Study the drawing (mm; zero at the part's minimum x, y, z) and answer. Give positions to 0.01 mm unless a question says otherwise; leave off trailing zeros. Order: outer loops, then holes, each group sorted by start corner. A loop starts at its lowest first (then second) coordinate and runs counter-clockwise, first axis right, second up. Notation, with made-up numbers: (14.25, 20.5) - (41.25, 20.5) arc R8 cw to (41.25, 31.5) - close; hole circle Ø6 at (89, 33.5). An arc over 180 degrees is marked (long way). Return JSON: item names as keys, results as strings.
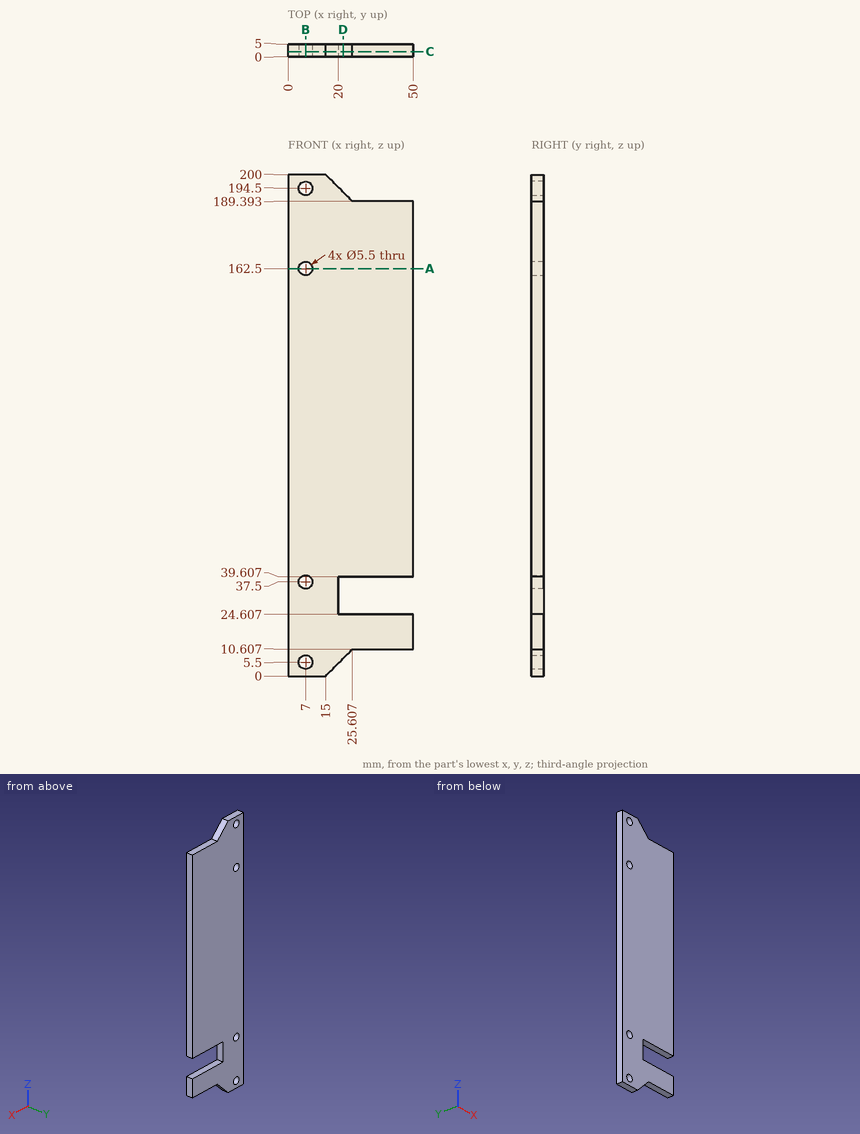
Q1. A cutting plane is placed at C-C (y = 2). Write down the section's boundary in (x, z).
Values:
{"outline": "(0, 0) - (15, 0) - (25.61, 10.61) - (50, 10.61) - (50, 24.61) - (20, 24.61) - (20, 39.61) - (50, 39.61) - (50, 189.39) - (25.61, 189.39) - (15, 200) - (0, 200) - close; hole circle Ø5.5 at (7, 5.5); hole circle Ø5.5 at (7, 37.5); hole circle Ø5.5 at (7, 162.5); hole circle Ø5.5 at (7, 194.5)"}
Q2. Given pin 1 (5 mm diameter, centred on x = 7, z = 5.5, fed in from +Y), flat-ended and moving along its own axis, determine where the tip first touches the part or whether it passes through.
Values:
{"pin 1": "passes through"}
Q3. A cutting plane is placed at A-A (z = 162.5). Write down the section's boundary in (x, y).
Values:
{"outline": "(0, 0) - (4.25, 0) - (4.25, 5) - (0, 5) - close; (9.75, 0) - (50, 0) - (50, 5) - (9.75, 5) - close"}
Q4. A cutting plane is placed at B-B (x = 7). Write down the section's boundary in (y, z).
Values:
{"outline": "(0, 0) - (5, 0) - (5, 2.75) - (0, 2.75) - close; (0, 8.25) - (5, 8.25) - (5, 34.75) - (0, 34.75) - close; (0, 40.25) - (5, 40.25) - (5, 159.75) - (0, 159.75) - close; (0, 165.25) - (5, 165.25) - (5, 191.75) - (0, 191.75) - close; (0, 197.25) - (5, 197.25) - (5, 200) - (0, 200) - close"}
Q5. Consider L1, parallel to Z at x = 37.5, y = 3.95; L2, parallel to X at y = 2.6, z = 37.5; L3, parallel to Z at x = 5, y = 3.15 (1 decimal). Determine where each line is inside the solid, lowest interval first.
Values:
{"L1": "z = 10.61 to 24.61, 39.61 to 189.39", "L2": "x = 0 to 4.25, 9.75 to 20", "L3": "z = 0 to 3.6, 7.4 to 35.6, 39.4 to 160.6, 164.4 to 192.6, 196.4 to 200"}
Q6. A cutting plane is placed at D-D (x = 22). Write down the section's boundary in (y, z), and give its area (3 significant figures).
Values:
{"outline": "(0, 7) - (5, 7) - (5, 24.61) - (0, 24.61) - close; (0, 39.61) - (5, 39.61) - (5, 193) - (0, 193) - close", "area": "855 mm²"}
